The model under review builds one solid part; all positions refer to its coordinate system, in mm. Face numbers are marked on the shaded views. A direction names the side the tool comes from. Coordinates: 2 decimals unless noted, no trailing zeros. Order: outer loops, then holes, each group sorted by start corner. A loop starts at its lowest first (then second) coordinate and runs counter-clockwise, first axis right, second up.
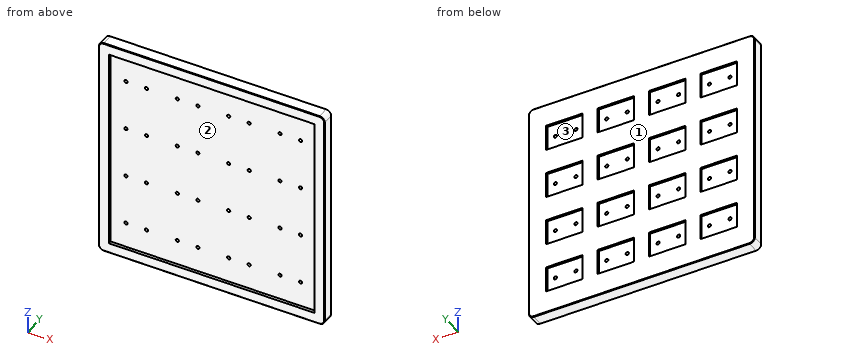
```python
from build123d import *

# Parameters (mm, degrees)
SKETCH1_W            = 220
SKETCH1_H            = 220
BOSS_EXTRUDE1_DEPTH  = 12
SKETCH2_W            = 35.5
SKETCH2_H            = 25.5
CUT_EXTRUDE1_DEPTH   = 2
LPATTERN1_COUNT      = 4
LPATTERN1_PITCH      = 50
LPATTERN1_COUNT_DIR2 = 4
LPATTERN1_PITCH_DIR2 = 50
SKETCH3_R            = 1.55
CUT_EXTRUDE2_DEPTH   = 312.287648325
LPATTERN2_COUNT      = 4
LPATTERN2_PITCH      = 50
LPATTERN2_COUNT_DIR2 = 4
LPATTERN2_PITCH_DIR2 = 50
SKETCH4_W            = 200
SKETCH4_H            = 200
CUT_EXTRUDE3_DEPTH   = 3
FILLET1_R            = 5
CHAMFER1_SIZE        = 0.5


with BuildPart() as part:
    # Sketch1 → Boss-Extrude1 (new body)
    with BuildSketch(Plane(origin=(0, 0, 0), x_dir=(1, 0, 0), z_dir=(0, 1, 0))):
        with Locations((110, 110)):
            Rectangle(SKETCH1_W, SKETCH1_H)
    extrude(amount=BOSS_EXTRUDE1_DEPTH)

    # Sketch2 → Cut-Extrude1 (cut)
    with BuildSketch(Plane(origin=(0, 12, 0), x_dir=(1, 0, 0), z_dir=(0, 1, 0))):
        with Locations((35, 35)):
            Rectangle(SKETCH2_W, SKETCH2_H)
    cut_extrude1 = extrude(amount=-CUT_EXTRUDE1_DEPTH, mode=Mode.SUBTRACT)

    # LPattern1: Cut-Extrude1 4 × 4
    with Locations(*[(j * LPATTERN1_PITCH_DIR2, 0, -i * LPATTERN1_PITCH) for i in range(LPATTERN1_COUNT) for j in range(LPATTERN1_COUNT_DIR2) if (i, j) != (0, 0)]):
        add(cut_extrude1, mode=Mode.SUBTRACT)

    # Sketch3 → Cut-Extrude2 (cut, through all)
    with BuildSketch(Plane(origin=(0, 10, 0), x_dir=(1, 0, 0), z_dir=(0, 1, 0))):
        with Locations(Location((25, 35, 0), (0, 0, 270))):
            Circle(SKETCH3_R)
        with Locations(Location((45, 35, 0), (0, 0, 270))):
            Circle(SKETCH3_R)
    cut_extrude2 = extrude(amount=-CUT_EXTRUDE2_DEPTH, mode=Mode.SUBTRACT)

    # LPattern2: Cut-Extrude2 4 × 4
    with Locations(*[(j * LPATTERN2_PITCH_DIR2, 0, -i * LPATTERN2_PITCH) for i in range(LPATTERN2_COUNT) for j in range(LPATTERN2_COUNT_DIR2) if (i, j) != (0, 0)]):
        add(cut_extrude2, mode=Mode.SUBTRACT)

    # Sketch4 → Cut-Extrude3 (cut)
    with BuildSketch(Plane.XZ):
        with Locations((110, -110)):
            Rectangle(SKETCH4_W, SKETCH4_H)
    extrude(amount=-CUT_EXTRUDE3_DEPTH, mode=Mode.SUBTRACT)

    # Fillet1
    fillet1_edges = [part.edges().sort_by_distance(p)[0] for p in [
        (0, 6, -220),
        (220, 6, -220),
        (220, 6, 0),
        (0, 6, 0),
    ]]
    fillet(fillet1_edges, radius=FILLET1_R)

    # Chamfer1
    chamfer1_edges = [part.edges().sort_by_distance(p)[0] for p in [
        (0, 0, -110),
        (0, 12, -110),
        (110, 0, -220),
        (220, 0, -110),
        (110, 0, 0),
        (218.535533906, 0, -218.535533906),
        (218.535533906, 0, -1.464466094),
        (1.464466094, 0, -1.464466094),
        (1.464466094, 0, -218.535533906),
        (110, 12, -220),
        (110, 12, 0),
        (220, 12, -110),
        (218.535533906, 12, -218.535533906),
        (218.535533906, 12, -1.464466094),
        (1.464466094, 12, -1.464466094),
        (1.464466094, 12, -218.535533906),
    ]]
    chamfer(chamfer1_edges, length=CHAMFER1_SIZE)


solid = part.part
```
(1) Machinability: for the marked faces 1, 2 and 3, which of the approach directions +Z, -Z, +X, -X, +Y, -Y give a long, thin tool a straight path to every point of the face, cutting with its end or side? Answer none if there is none.
A:
face 1: +Z, -Z, +X, -X, +Y
face 2: -Y
face 3: +Y
(2) Wall thickness on probe 1 along Z at (x, y) = (95, 7); probe 2 along Z at (x, y) = (82, 10.5); probe 3 along Z at (x, y) = (15, 2): over which ranges is each line inside the solid? List them lowest first.
A:
probe 1: z = -220 to -186.55, -183.45 to -136.55, -133.45 to -86.55, -83.45 to -36.55, -33.45 to 0
probe 2: z = -220 to -197.75, -172.25 to -147.75, -122.25 to -97.75, -72.25 to -47.75, -22.25 to 0
probe 3: z = -220 to -210, -10 to 0
(3) We need section A-A, the plane z = -115. Write out the cut boundary in (x, y), and give its area (3 significant figures).
A:
outline: (0, 0.5) - (0.5, 0) - (10, 0) - (10, 3) - (210, 3) - (210, 0) - (219.5, 0) - (220, 0.5) - (220, 11.5) - (219.5, 12) - (0.5, 12) - (0, 11.5) - close
area: 2,040 mm2
(4) For pin 1 Ø13 at (x, z) = (87.5, -133) entering from +Y; pin 2 Ø3.5 at (x, z) = (125, -85) entering from -Y, all flat-tipped, find the tip position at first contact; note any pin that passes through.
A:
pin 1: stops at y = 10
pin 2: stops at y = 3
(5) We need section B-B, the plane x = 185. Write out the cut boundary in (y, z).
A:
outline: (0, -219.5) - (0.5, -220) - (11.5, -220) - (12, -219.5) - (12, -197.75) - (10, -197.75) - (10, -172.25) - (12, -172.25) - (12, -147.75) - (10, -147.75) - (10, -122.25) - (12, -122.25) - (12, -97.75) - (10, -97.75) - (10, -72.25) - (12, -72.25) - (12, -47.75) - (10, -47.75) - (10, -22.25) - (12, -22.25) - (12, -0.5) - (11.5, 0) - (0.5, 0) - (0, -0.5) - (0, -10) - (3, -10) - (3, -210) - (0, -210) - close
